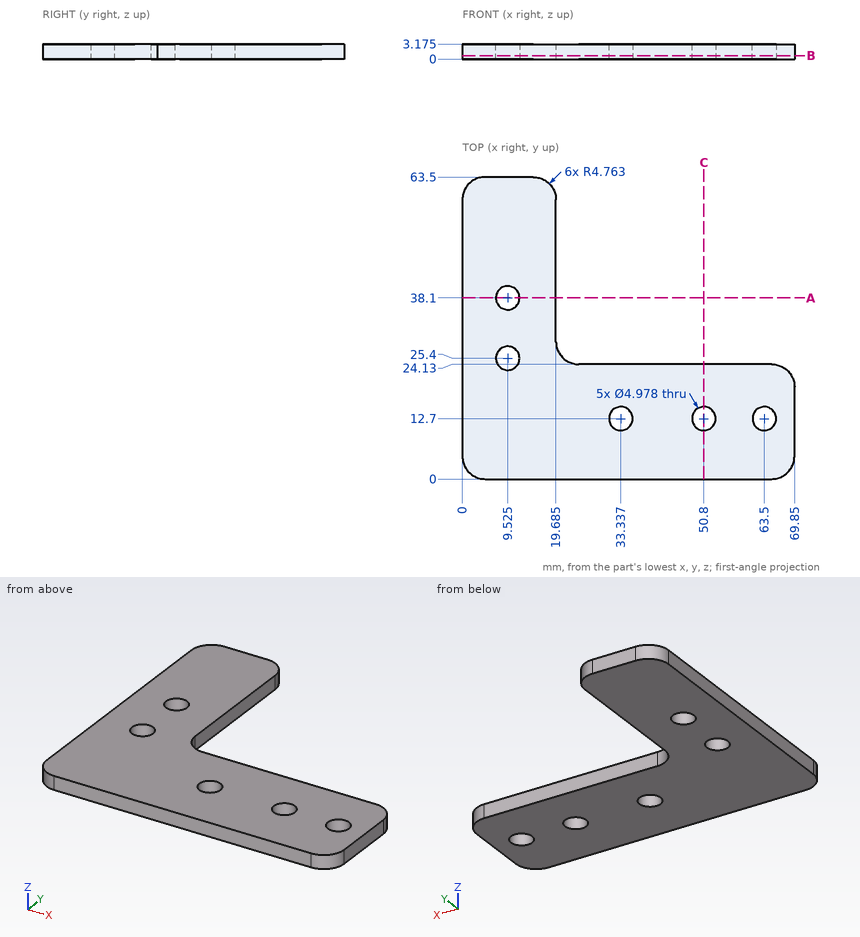
Geometry check sheet. Reference: drawing and pictorial views, mm from the part's lowest x, y, z. Round coordinates to 2 decimals unless told otherwise and drop trailing zeros. Loops run counter-clockwise (first coordinate to the right, second up) from the corner with the lowest first, then second, coordinate; pieces in that order, holes last. Notation, with made-up numbers: (82.5, 71) -> (109.5, 71) arc R18 ccw to (109.5, 85) -> close; hole circle Ø4 at (72, -18.5). An arc over 180 degrees is marked (long way). Answer as a JSON object with one key per item and string values. Group by question number.
Item 1: Depth check by flat-ended pin: pin 1 Ø1.6 at (x, z) = (50, 1.5) entering from +Y; pin 2 Ø8 at (x, y) = (50.8, 12.7) entering from +Z (1 decimal); pin 3 Ø1 at (y, z) = (38, 1.5) entering from +X (1 decimal). Enter the tip coordinate at first touch or a pass-through.
Item 2: Thickness scan on line 1 along Y through (x, z) = (63.5, 1.45); line 2 along X through (y, z) = (49, 1.7) (1 decimal); line 3 along Y through (x, z) = (29.5, 0.55). Record the ranges inside material, lowest first.
Item 3: Cross-section at C-C, the plane x = 50.8. Record the cut outline in (y, z) (1 decimal).
Item 4: Cross-section at A-A, the plane y = 38.1. Record the cut outline in (x, z) (1 decimal), plus the area to 3 significant figures.
Item 5: Cross-section at B-B, the plane z = 0.75. Count the separate pieces of the cut face and the enclosed holes in it, plus the area to 3 significant figures.
Determined:
{
 "1": {"pin 1": "stops at y = 24.13", "pin 2": "stops at z = 3.2", "pin 3": "stops at x = 19.7"},
 "2": {"line 1": "y = 0 to 10.21, 15.19 to 24.13", "line 2": "x = 0 to 19.7", "line 3": "y = 0 to 24.13"},
 "3": {"outline": "(0, 0) -> (10.2, 0) -> (10.2, 3.2) -> (0, 3.2) -> close; (15.2, 0) -> (24.1, 0) -> (24.1, 3.2) -> (15.2, 3.2) -> close"},
 "4": {"outline": "(0, 0) -> (7, 0) -> (7, 3.2) -> (0, 3.2) -> close; (12, 0) -> (19.7, 0) -> (19.7, 3.2) -> (12, 3.2) -> close", "area": "46.7 mm²"},
 "5": {"separate pieces": "1", "enclosed holes": "5", "area": "2,340 mm²"}
}
